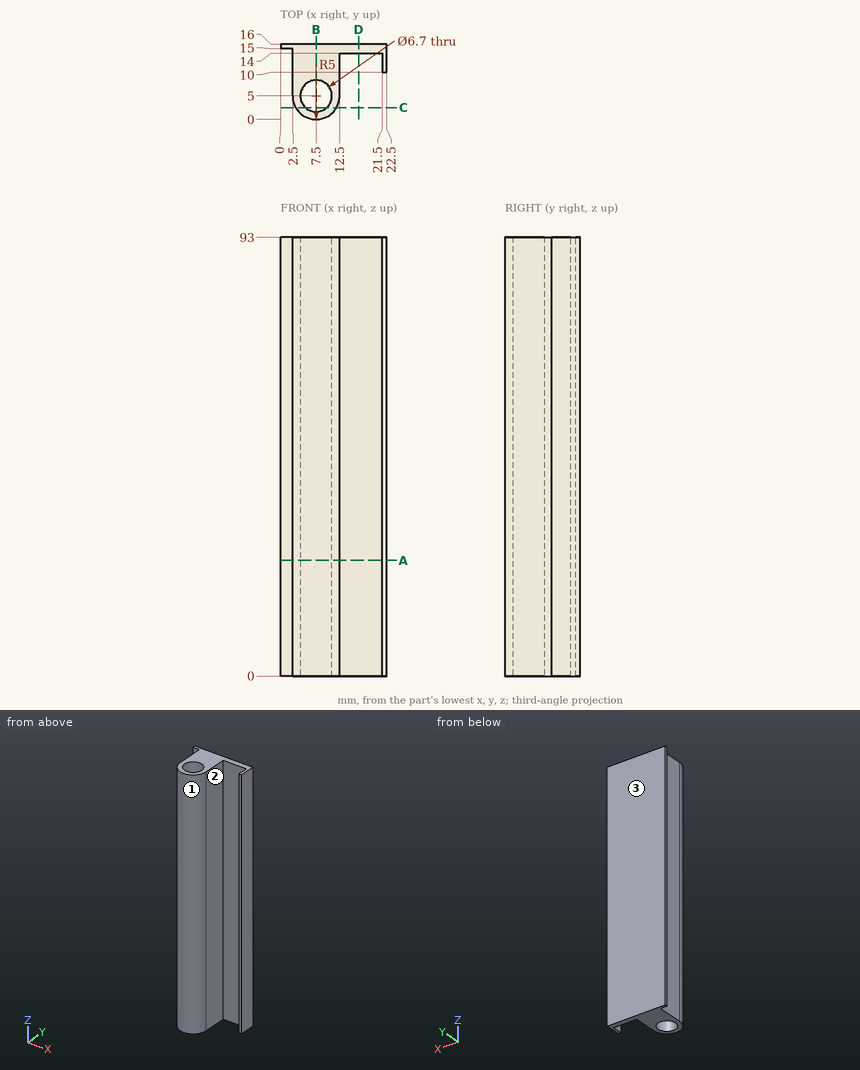
Print and shaded views of the part. All mm, measured from the part's lowest x, y and z. Round coordinates to 2 decimals unless told otherwise and drop trailing zeros. Loops run counter-clockwise (first coordinate to the right, second up) from the corner with the lowest first, then second, coordinate; pieces in that order, holes last. Notation, with made-up numbers: (81.25, 23) -> (95.25, 23) arc R33 ccw to (95.25, 52) -> close; hole circle Ø4 at (37, 58.25). An arc over 180 degrees is marked (long way). Use CSV: the item, a comma, the result in double quotes. Start each with the question number.
1) Cut at A-A, the plane z = 24.5. Write the cut outline in (x, y), plus the area to 3 significant figures.
2) Cut at D-D, the plane x = 16.5. Write the cut outline in (y, z).
3) Cut at B-B, the plane x = 7.5. Write the cut outline in (y, z), plus the area to 3 significant figures.
4) Drop flat-ended pins along their axis: P1, Ø1.5, axis at y = 5, z = 46, coming from the +X side; P2, Ø2, axis at y = 13.5, z = 43, coming from the -X side; P3, Ø1.5, axis at x = 19.5, z = 39.5, coming from the -Y side. Give the stop position or say it passes through.
5) Wall check: L1, parallel to X at y = 11.5, z = 57; L2, parallel to Y at x = 7.5, z = 63; L3, parallel to Y at x = 15.5, z = 87. Give the ranges that are in metal, low to high. Write a range as [from, to].
6) Cut at C-C, the plane y = 2.5. Write the cut outline in (x, z).
7) Pull direction X, two halves, no side cores. Call the marked faces 1, 2 and 3: +X half, -X half, draft (parallel to the pull), parting line (faces both ways), or undercut.
Determined:
1,outline,"(0, 15) -> (2.5, 15) -> (2.5, 5) arc R5 ccw to (12.5, 5) -> (12.5, 14) -> (21.5, 14) -> (21.5, 10) -> (22.5, 10) -> (22.5, 16) -> (0, 16) -> close; hole circle Ø6.7 at (7.5, 5)"
1,area,"141 mm2"
2,outline,"(14, 0) -> (16, 0) -> (16, 93) -> (14, 93) -> close"
3,outline,"(0, 0) -> (1.65, 0) -> (1.65, 93) -> (0, 93) -> close; (8.35, 0) -> (16, 0) -> (16, 93) -> (8.35, 93) -> close"
3,area,"865 mm2"
4,P1,"stops at x = 12.5"
4,P2,"stops at x = 2.5"
4,P3,"stops at y = 14"
5,L1,"x = [2.5, 12.5], [21.5, 22.5]"
5,L2,"y = [0, 1.65], [8.35, 16]"
5,L3,"y = [14, 16]"
6,outline,"(3.17, 0) -> (5.27, 0) -> (5.27, 93) -> (3.17, 93) -> close; (9.73, 0) -> (11.83, 0) -> (11.83, 93) -> (9.73, 93) -> close"
7,face 1,"parting line"
7,face 2,"undercut"
7,face 3,"draft"
